Source: CAD feature listing. Evaluate the final solid. Frame: model axes, mm. A direction names the side the tool comes from. Round coordinates to 2 decimals unless told otherwise and drop trailing zeros. Order: outer loops, then holes, each group sorted by start corner. A loop starts at its lowest first (then second) coordinate and runs counter-clockwise, first axis right, second up. Notation, with made-up numbers: M -19.5,-0.75 L 33.5,-0.75 A33 ccw 33.5,30.25 Z; hole C 26.5,72 d2. An arc over 180 degrees is marked long. Use one line per item in the form item = value. Start each with the question number.
Q1. Pull-direction query (Y, two-part tool) for faces 5 (the flat face through (1, -5.08, -37)), 6 (the flat face through (0, 6.35, -18)), 7 (the flat face through (0, -6, -38.1)), 8 (the flat face through (0.018, 2.576, -28.289)); classes: pulls with the +Y half, pulls with the -Y half, needs draft (parallel to the pull), parting line crosses it, or undercut.
Q2. Section B-B (z = -20). Return the cut outline in (x, y), plus the area to 3 significant figures.
Q3. Reachability of faces 1 (the flat face through (1, 5.08, -37)), 2 (the cylindrical face through (-0.22, -5.724, -37.314)), 3 (the cylindrical face through (-0.15, -5.83, -11.48)), 4 (the flat face through (0.02, 2.99, -9.54)) from +Z, -Z, +X, -X, +Y, -Y: full face, straight path, thin tool, end or side. Return the list, or none.
Q4. Section D-D (z = -34.5). Return the cut outline in (x, y).
Q5. Section A-A (x = 0). Give the number of separate pieces and of enclosed holes in the cut face, plus the area to 3 significant figures.
Q6. Material intervals for probe 1 along Y at (x, z) = (-0.55, -31); probe 2 along Y at (x, z) = (0.1, -25); probe 3 along Y at (x, z) = (0.75, -2), sorted ascending.
Q7. Section C-C (y = -2.5). Return the cut outline in (x, z), plus the area to 3 significant figures.
from build123d import *

# Parameters (mm, degrees)
F1_DEPTH = 6.35
F3_DEPTH = 2.54
F4_W     = 10.16
F4_H     = 2.9410431877
F5_DEPTH = 2.54
F6_R     = 1.016
F7_DEPTH = 12.7
F8_R     = 1.1176
F9_DEPTH = 2.54


# Not quite as in the source:
# - a feature names something its author has since deleted; it is built from what else it names


with BuildPart() as f1:
    # F0 (on Front) → F1 (new body, symmetric)
    with BuildSketch(Plane.XZ):
        with BuildLine():
            Line((1.27, -38.1), (1.27, 0))
            ThreePointArc((1.27, 0), (0.8980256121, 0.8980256121), (0, 1.27))
            ThreePointArc((0, 1.27), (-0.8980256121, 0.8980256121), (-1.27, 0))
            Line((-1.27, 0), (-1.27, -38.1))
            Line((-1.27, -38.1), (1.27, -38.1))
        make_face()
    extrude(amount=F1_DEPTH, both=True)

    # F2 (on face) → F3 (cut)
    with BuildSketch(Plane.YZ.offset(1.27)):
        Polygon((0.635, -19.4826158311), (5.2897260698, -32.2506076148), (5.2897260698, -6.7146240474), align=None)
        Polygon((0, -35.1589568123), (5.08, -35.1589568123), (0, -21.2244314957), align=None)
        Polygon((0, -1.0980047432), (0, -17.7408001665), (6.067332674, -1.0980047432), align=None)
        Polygon((-6.067332674, -1.0980047432), (0, -17.7408001665), (0, -1.0980047432), align=None)
        Polygon((0, -35.1589568123), (0, -21.2244314957), (-5.08, -35.1589568123), align=None)
        Polygon((-5.2897260698, -32.2506076148), (-0.635, -19.4826158311), (-5.2897260698, -6.7146240474), align=None)
    extrude(amount=-F3_DEPTH, mode=Mode.SUBTRACT)

    # F4 (on face) → F5 (cut)
    with BuildSketch(Plane.YZ.offset(1.27)):
        with Locations((0, -36.6294784061)):
            Rectangle(F4_W, F4_H)
    extrude(amount=-F5_DEPTH, mode=Mode.SUBTRACT)

    # F6 (on face) → F7 (cut)
    with BuildSketch(Plane.XZ.offset(6.35)):
        with Locations((0, -36.322)):
            Circle(F6_R)
        Circle(F6_R)
    extrude(amount=-F7_DEPTH, mode=Mode.SUBTRACT)

    # F8 (on face) → F9 (cut)
    with BuildSketch(Plane.XZ.offset(6.35)):
        with Locations((0, -12.589443475)):
            Circle(F8_R)
    extrude(amount=-F9_DEPTH, mode=Mode.SUBTRACT)


solid = f1.part
Results list:
q1.face_5 = undercut
q1.face_6 = pulls with the +Y half
q1.face_7 = needs draft
q1.face_8 = undercut
q2.outline = M -1.27,-6.35 L 1.27,-6.35 L 1.27,-5.29 L -1.27,-5.29 Z; M -1.27,-0.82 L 1.27,-0.82 L 1.27,0.82 L -1.27,0.82 Z; M -1.27,5.29 L 1.27,5.29 L 1.27,6.35 L -1.27,6.35 Z
q2.area = 9.57 mm2
q3.face_1 = -Z, +X, -X
q3.face_2 = +Y, -Y
q3.face_3 = -Y
q3.face_4 = +X, -X
q4.outline = M -1.27,-6.35 L 1.27,-6.35 L 1.27,-4.84 L -1.27,-4.84 Z; M -1.27,4.84 L 1.27,4.84 L 1.27,6.35 L -1.27,6.35 Z
q5.separate_pieces = 4
q5.enclosed_holes = 2
q5.area = 146 mm2
q6.probe_1 = -6.35 to -5.29, -4.83 to -3.56, 3.56 to 4.83, 5.29 to 6.35
q6.probe_2 = -6.35 to -5.29, -2.65 to -1.38, 1.38 to 2.65, 5.29 to 6.35
q6.probe_3 = -6.35 to -5.74, 5.74 to 6.35
q7.outline = M -1.27,-28.08 L 1.27,-28.08 L 1.27,-24.6 L -1.27,-24.6 Z; M -1.27,-14.37 L 1.27,-14.37 L 1.27,-10.88 L -1.27,-10.88 Z; M -1.27,-1.1 L 1.27,-1.1 L 1.27,0 A1.27 ccw -1.27,0 Z; hole C 0,0 d2.03
q7.area = 19.8 mm2
